from build123d import *

# Parameters (mm, degrees)
F0_W     = 1371.6
F0_H     = 1772.92
F2_DEPTH = 1701.8
F3_W     = 736.6
F3_H     = 83.82
F4_DEPTH = 1701.8
F6_DEPTH = 1701.8
F7_R     = 80.01
F8_DEPTH = 317.5


with BuildPart() as f2:
    # F0 (on Front) → F2 (new body)
    with BuildSketch(Plane.XZ):
        with Locations((641.200314182, 852.594570539)):
            Rectangle(F0_W, F0_H)
    extrude(amount=F2_DEPTH)

    # F3 (on face) → F4 (cut)
    with BuildSketch(Plane.XZ.offset(1701.8)):
        with Locations((958.700314182, 1379.644570539)):
            Rectangle(F3_W, F3_H)
    extrude(amount=-F4_DEPTH, mode=Mode.SUBTRACT)

    # F5 (on face) → F6 (cut)
    with BuildSketch(Plane.XZ.offset(1701.8)):
        with BuildLine():
            ThreePointArc((1059.1441740484, 410.634570539), (1107.3561179491, 527.0284993725), (1123.800314182, 651.934570539))
            ThreePointArc((1123.800314182, 651.934570539), (1107.3561179491, 776.8406417055), (1059.1441740484, 893.234570539))
            Line((1059.1441740484, 893.234570539), (692.000314182, 893.234570539))
            Line((692.000314182, 893.234570539), (692.000314182, 410.634570539))
            Line((692.000314182, 410.634570539), (1059.1441740484, 410.634570539))
        make_face()
        with BuildLine():
            ThreePointArc((1059.1441740484, 893.234570539), (1107.3561179491, 776.8406417055), (1123.800314182, 651.934570539))
            ThreePointArc((1123.800314182, 651.934570539), (1107.3561179491, 527.0284993725), (1059.1441740484, 410.634570539))
            Line((1059.1441740484, 410.634570539), (1327.000314182, 410.634570539))
            Line((1327.000314182, 410.634570539), (1327.000314182, 893.234570539))
            Line((1327.000314182, 893.234570539), (1059.1441740484, 893.234570539))
        make_face()
        with BuildLine():
            Line((692.000314182, 893.234570539), (1059.1441740484, 893.234570539))
            ThreePointArc((1059.1441740484, 893.234570539), (158.600314182, 651.934570539), (1059.1441740484, 410.634570539))
            Line((1059.1441740484, 410.634570539), (692.000314182, 410.634570539))
            Line((692.000314182, 410.634570539), (692.000314182, 893.234570539))
        make_face()
    extrude(amount=-F6_DEPTH, mode=Mode.SUBTRACT)

    # F7 (on face) → F8 (cut)
    with BuildSketch(Plane.XY.offset(1739.054570539)):
        with Locations((1116.180314182, -850.9)):
            Circle(F7_R)
    extrude(amount=-F8_DEPTH, mode=Mode.SUBTRACT)


solid = f2.part
Geometry: final body of the model. Coordinates: model frame, mm. A direction names the side the tool comes from. Give positions to 0.01 mm unless a question says otherwise; leave off trailing zeros. Loops run counter-clockwise (first coordinate to the right, second up) from the corner with the lowest first, then second, coordinate; pieces in that order, holes last. Notation, with made-up numbers: M 15,62.5 L 22,62.5 A17 cw 22,86.5 Z; hole C -28,-27 d3. An arc over 180 degrees is marked long. Put each result on its own line as item: value.
1) Cut plane A-A, the plane y = -850.9. Return the cut outline in (x, z), plus the area to 3 significant figures.
Computed values:
outline: M -44.6,-33.87 L 1327,-33.87 L 1327,410.63 L 1059.14,410.63 A482.6 cw long 1059.14,893.23 L 1327,893.23 L 1327,1337.73 L 590.4,1337.73 L 590.4,1421.55 L 1036.17,1421.55 L 1036.17,1739.05 L -44.6,1739.05 Z; M 1196.19,1421.55 L 1327,1421.55 L 1327,1739.05 L 1196.19,1739.05 Z
area: 1,480,000 mm^2
2) Cut plane D-D, the plane y = -1401. Return the cut outline in (x, z).
Computed values:
outline: M -44.6,-33.87 L 1327,-33.87 L 1327,410.63 L 1059.14,410.63 A482.6 cw long 1059.14,893.23 L 1327,893.23 L 1327,1337.73 L 590.4,1337.73 L 590.4,1421.55 L 1327,1421.55 L 1327,1739.05 L -44.6,1739.05 Z
3) Material intervals for L1, parallel to Z at x = 1262, y = -129; L2, parallel to Z at x = 630, y = -1117; L3, parallel to X at y = -728.5, z = 636.5, sorted ascending. Write a range as from..to.
Computed values:
L1: z = -33.87..410.63, 893.23..1337.73, 1421.55..1739.05
L2: z = -33.87..169.46, 1134.4..1337.73, 1421.55..1739.05
L3: x = -44.6..158.85
4) Mould query, pull axis X, two halves, no side actions, for faces 1 (the flat face through (632, -839, -33.865)), 2 (the cylindrical face through (1098.8, -929, 1582.5)), 3 (the flat face through (1327, -839, 1112)). Classes: released by +X, released by -X, zero draft, split by the parting line, or undercut.
Computed values:
face 1: zero draft
face 2: undercut
face 3: released by +X
5) Cut plane C-C, the plane x = 340.5. Return the cut outline in (y, z).
Computed values:
outline: M -1701.8,-33.87 L 0,-33.87 L 0,274.47 L -1701.8,274.47 Z; M -1701.8,1029.4 L 0,1029.4 L 0,1739.05 L -1701.8,1739.05 Z
6) Reachability of faces 4 (the flat face through (1327, -839, 185)), 5 (the flat face through (590.4, -863, 1379)) from +Z, -Z, +X, -X, +Y, -Y: full face, straight path, thin tool, end or side. Return the list, or none.
Computed values:
face 4: +Z, -Z, +X, +Y, -Y
face 5: +X, +Y, -Y
7) Cut plane B-B, the plane z = 277.5. Return the cut outline in (x, y).
Computed values:
outline: M -44.6,-1701.8 L 336.73,-1701.8 L 336.73,0 L -44.6,0 Z; M 945.67,-1701.8 L 1327,-1701.8 L 1327,0 L 945.67,0 Z
